from build123d import *

# Parameters (mm, degrees)
CROQUIS1_R              = 7.5
SALIENTE_EXTRUIR1_DEPTH = 30
SALIENTE_EXTRUIR2_DEPTH = 4
SALIENTE_EXTRUIR3_DEPTH = 5
CROQUIS4_R              = 1.5
CORTAR_EXTRUIR1_DEPTH   = 5
CROQUIS5_R              = 5
CORTAR_EXTRUIR2_DEPTH   = 57.644348631


with BuildPart() as part:
    # Croquis1 → Saliente-Extruir1 (new body)
    with BuildSketch(Plane(origin=(0, 0, 0), x_dir=(1, 0, 0), z_dir=(0, 1, 0))):
        with Locations(Location((-15.184301915, -1.03253253, 0), (0, 0, 270))):
            Circle(CROQUIS1_R)
    extrude(amount=SALIENTE_EXTRUIR1_DEPTH)

    # Croquis2 → Saliente-Extruir2 (add)
    with BuildSketch(Plane(origin=(0, 30, 0), x_dir=(1, 0, 0), z_dir=(0, 1, 0))):
        with BuildLine():
            Line((-15.589707321, -8.521567612), (-34.035653267, -7.523029601))
            ThreePointArc((-34.035653267, -7.523029601), (-40.184301915, -1.03253253), (-34.035653267, 5.457964541))
            Line((-34.035653267, 5.457964541), (-15.589707321, 6.456502552))
            ThreePointArc((-15.589707321, 6.456502552), (-7.684301915, -1.03253253), (-15.589707321, -8.521567612))
        make_face()
    extrude(amount=SALIENTE_EXTRUIR2_DEPTH)

    # Croquis3 → Saliente-Extruir3 (add)
    with BuildSketch(Plane(origin=(0, 0, 0), x_dir=(-1, 0, 0), z_dir=(0, -1, 0))):
        with BuildLine():
            Line((32.028051915, -5.452723243), (16.590551915, -8.399517052))
            ThreePointArc((16.590551915, -8.399517052), (7.684301915, -1.03253253), (16.590551915, 6.334451991))
            Line((16.590551915, 6.334451991), (32.028051915, 3.387658183))
            ThreePointArc((32.028051915, 3.387658183), (35.684301915, -1.03253253), (32.028051915, -5.452723243))
        make_face()
    extrude(amount=SALIENTE_EXTRUIR3_DEPTH)

    # Croquis4 → Cortar-Extruir1 (cut)
    with BuildSketch(Plane(origin=(0, 34, 0), x_dir=(1, 0, 0), z_dir=(0, 1, 0))):
        with Locations(Location((-33.684301915, -1.03253253, 0), (0, 0, 270))):
            Circle(CROQUIS4_R)
    extrude(amount=-CORTAR_EXTRUIR1_DEPTH, mode=Mode.SUBTRACT)

    # Croquis5 → Cortar-Extruir2 (cut, through all)
    with BuildSketch(Plane(origin=(0, 34, 0), x_dir=(1, 0, 0), z_dir=(0, 1, 0))):
        with Locations(Location((-15.184301915, -1.03253253, 0), (0, 0, 270))):
            Circle(CROQUIS5_R)
    extrude(amount=-CORTAR_EXTRUIR2_DEPTH, mode=Mode.SUBTRACT)


solid = part.part
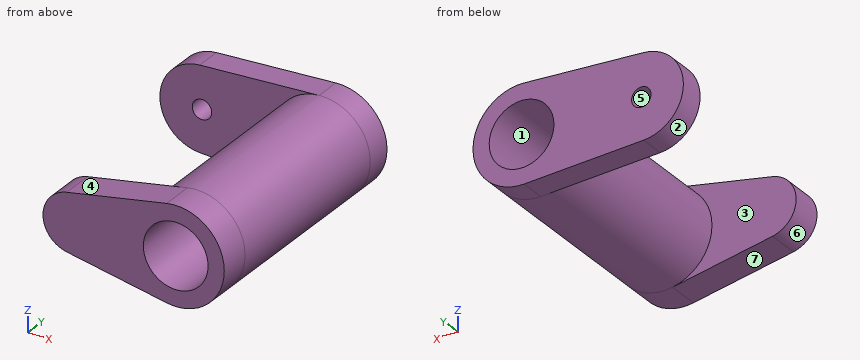
Verification items for the finished model (mm, model axes). Face numbers are marked on the shaded views. A direction names the side the tool comes from. Coordinates: 2 decimals unless noted, no trailing zeros. Order: outer loops, then holes, each group sorted by start corner. A loop starts at its lowest first (then second) coordinate and runs counter-clockwise, first axis right, second up.
1. Scan lines: line 1 (Y direction, x = -31.5, z = 3); line 2 (Y direction, x = -34.5, z = 1); line 3 (Z direction, x = -18, y = 28.5). Record each from-to range of solid material in increasing order.
Results found:
line 1: y = -5 to 0, 30 to 34
line 2: y = -5 to 0
line 3: z = -5.92 to -3.1, 5.16 to 7.98
2. Sectioned sample at B-B, the plane x = -19.5. Record the cut outline in (y, z).
Results found:
outline: (-5, -5.78) - (0, -5.78) - (0, -5.1) - (30, -5.1) - (30, -6.24) - (34, -6.24) - (34, -1.49) - (-5, -1.49) - close; (-5, 3.56) - (34, 3.56) - (34, 8.31) - (30, 8.31) - (30, 7.17) - (0, 7.17) - (0, 7.84) - (-5, 7.84) - close
3. Set-up check for the marked faces 4, 5, 6 and 7: record each of +Z, -Z, +X, -X, +Y, -Y from which the full face is reachable in a straight line by a thin tool's end or side.
Results found:
face 4: +Z, -X, -Y
face 5: +Y
face 6: -X, -Y
face 7: -Z, -X, -Y
4. Release check for a two-part mould opening along Z. For the marked faces 1, 2 and 3 record: +Z half, -Z half, draft (parallel to the pull), parting line (faces both ways), or undercut.
Results found:
face 1: undercut
face 2: parting line
face 3: draft
5. Sectioned sample at A-A, the plane z = 1.5. Record the cut outline in (x, y).
Results found:
outline: (-40.17, 30) - (-35.11, 30) - (-35.11, 34) - (-40.17, 34) - close; (-35.66, -5) - (-20.16, -5) - (-20.16, 34) - (-32.26, 34) - (-32.26, 30) - (-22.67, 30) - (-22.67, 0) - (-35.66, 0) - close; (-10.21, -5) - (-7.7, -5) - (-7.7, 34) - (-10.21, 34) - close
6. Sectioned sample at C-C, the plane y = -1.5. Record the cut outline in (x, z), and give its area (3 significant figures).
Results found:
outline: (-32.03, -3.39) - (-16.59, -6.33) arc R7.5 ccw (long way) to (-16.59, 8.4) - (-32.03, 5.45) arc R4.5 ccw to start; hole circle Ø10 at (-15.18, 1.03)
area: 237 mm2
7. Sectioned sample at D-D, the plane z = 4.5. Record the cut outline in (x, y).
Results found:
outline: (-39.18, 30) - (-21.83, 30) - (-21.83, 0) - (-34.05, 0) - (-34.05, -5) - (-18.79, -5) - (-18.79, 34) - (-39.18, 34) - close; (-11.58, -5) - (-8.53, -5) - (-8.53, 34) - (-11.58, 34) - close
8. Go/stop test with flat-tipped pins: pin 1 Ø1 at (y, z) = (21.5, 5) entering from +X; pin 2 Ø1.5 at (y, z) = (18.5, -4.5) entering from -X; pin 3 Ø3.5 at (x, z) = (-33.68, 1.03) entering from +Y; pin 4 Ø3 at (y, z) = (2, 5) entering from -X. Record where each tip stops, or that it passes through.
Results found:
pin 1: stops at x = -8.53
pin 2: stops at x = -20.96
pin 3: stops at y = 34
pin 4: stops at x = -22.27
